Verification items for the finished model (mm, model axes). A direction names the side the tool comes from. Round coordinates to 2 decimals unless told otherwise and drop trailing zeros. Write each loop counter-clockwise with the first axis right and the second up, starting at its lowest first coordinate (ties: lowest second). Pieces come first, ordered by that corner, then holes. Notation, with made-up numbers: (44.25, -35) - (90.25, -35) arc R20 cw to (90.25, -20) - close; hole circle Ø9 at (30.25, 74). An arc over 180 degrees is marked (long way). Write each question's results on one line, items separated by ' | '.
```python
from build123d import *

# Parameters (mm, degrees)
SKETCH1_R           = 10
BOSS_EXTRUDE1_DEPTH = 15
SKETCH2_W           = 21
SKETCH2_H           = 21
BOSS_EXTRUDE2_DEPTH = 3
SKETCH3_R           = 1
BOSS_EXTRUDE3_DEPTH = 2.5
SKETCH4_W           = 3
SKETCH4_H           = 5
CUT_EXTRUDE1_DEPTH  = 3.5


with BuildPart() as part:
    # Sketch1 → Boss-Extrude1 (new body)
    with BuildSketch(Plane.XY):
        Circle(SKETCH1_R)
    extrude(amount=BOSS_EXTRUDE1_DEPTH)

    # Sketch2 → Boss-Extrude2 (add)
    with BuildSketch(Plane(origin=(0, 0, 0), x_dir=(-1, 0, 0), z_dir=(0, 0, -1))):
        Rectangle(SKETCH2_W, SKETCH2_H)
    extrude(amount=BOSS_EXTRUDE2_DEPTH)

    # Sketch3 → Boss-Extrude3 (add, symmetric)
    with BuildSketch(Plane(origin=(0, 0, 0), x_dir=(0, 0, -1), z_dir=(1, 0, 0))):
        with BuildLine():
            Line((-15, 2.5), (-15, -2.5))
            Line((-15, -2.5), (-17, -2.5))
            ThreePointArc((-17, -2.5), (-19.5, 0), (-17, 2.5))
            Line((-17, 2.5), (-15, 2.5))
        make_face()
        with Locations((-17, 0)):
            Circle(SKETCH3_R, mode=Mode.SUBTRACT)
    extrude(amount=BOSS_EXTRUDE3_DEPTH, both=True)

    # Sketch4 → Cut-Extrude1 (cut)
    with BuildSketch(Plane.XY.offset(19.5)):
        Rectangle(SKETCH4_W, SKETCH4_H)
    extrude(amount=-CUT_EXTRUDE1_DEPTH, mode=Mode.SUBTRACT)


solid = part.part
```
(1) Section check A-A (x = 0). Record the cut outline in (y, z).
Answer:
outline: (-10.5, -3) - (10.5, -3) - (10.5, 0) - (10, 0) - (10, 15) - (2.5, 15) - (2.5, 16) - (-2.5, 16) - (-2.5, 15) - (-10, 15) - (-10, 0) - (-10.5, 0) - close
(2) Mould release check, pull along Z, two halves, no side actions. Record for faces 5 (the cylindrical face through (-2, 0, 16)), 6 (the flat face through (10.5, 0, -1)), 7 (the cylindrical face through (2, -0.1, 19.5)): released by +Z, released by -Z, zero draft, split by the parting line, or undercut.
Answer:
face 5: undercut | face 6: zero draft | face 7: released by +Z
(3) Thickness scan on L1, parallel to Z at x = -2, y = 0; L2, parallel to Y at x = 1.95, z = 17; L3, parallel to Z at x = -7, y = 6.25. Record the ranges inside material, lowest first.
Answer:
L1: -3 to 16, 18 to 19.5 | L2: -2.5 to -1, 1 to 2.5 | L3: -3 to 15
(4) Section check D-D (x = 8.5). Record the cut outline in (y, z).
Answer:
outline: (-10.5, -3) - (10.5, -3) - (10.5, 0) - (5.27, 0) - (5.27, 15) - (-5.27, 15) - (-5.27, 0) - (-10.5, 0) - close
(5) Set-up check for faces 1 (the flat face through (-1.5, 0, 18.2)), 2 (the flat face through (0, -4, 15)), 3 (the flat face through (2.5, 1.15, 17.22)), 4 (the flat face through (-2.5, 1.15, 17.22)): record each of +Z, -Z, +X, -X, +Y, -Y from which the full face is reachable in a straight line by a thin tool's end or side.
Answer:
face 1: +Z, +Y, -Y | face 2: +Z | face 3: +Z, +X, +Y, -Y | face 4: +Z, -X, +Y, -Y
(6) Section check B-B (y = 3.75). Record the cut outline in (x, z).
Answer:
outline: (-10.5, -3) - (10.5, -3) - (10.5, 0) - (9.27, 0) - (9.27, 15) - (-9.27, 15) - (-9.27, 0) - (-10.5, 0) - close
(7) Section check C-C (z = 1.5). Record the cut outline in (x, y), plus the area to 3 significant figures.
Answer:
outline: circle Ø20 at (0, 0) | area: 314 mm2
(8) Go/stop test with flat-tipped pins: pin 1 Ø6.5 at (x, y) = (-0.5, -4.5) entering from +Z; pin 2 Ø10 at (x, y) = (-3.5, -4) entering from +Z; pin 3 Ø2.5 at (y, z) = (0, 17) entering from +X; pin 4 Ø1 at (y, z) = (0.5, 18) entering from -X. Record where each tip stops, or that it passes through.
Answer:
pin 1: z = 19.07 | pin 2: z = 19.5 | pin 3: x = 2.5 | pin 4: x = -2.5
